from build123d import *

# Parameters (mm, degrees)
F0_R     = 43.75
F0_R_2   = 5
F1_DEPTH = 16
F2_R     = 7.5
F2_R_2   = 5
F3_DEPTH = 2.5
F4_R     = 39.3
F4_R_2   = 36.5
F4_R_3   = 32.8
F4_R_4   = 30
F5_DEPTH = 2.75
F6_SIZE  = 0.5


with BuildPart() as f1:
    # F0 (on Front) → F1 (new body)
    with BuildSketch(Plane.XZ):
        Circle(F0_R)
        Circle(F0_R_2, mode=Mode.SUBTRACT)
    extrude(amount=F1_DEPTH)

    # F2 (on face) → F3 (join)
    with BuildSketch(Plane.XZ.offset(16)):
        Circle(F2_R)
        Circle(F2_R_2, mode=Mode.SUBTRACT)
    extrude(amount=F3_DEPTH)

    # F4 (on face) → F5 (cut)
    with BuildSketch(Plane(origin=(0, 0, 0), x_dir=(-1, 0, 0), z_dir=(0, 1, 0))):
        Circle(F4_R)
        Circle(F4_R_2, mode=Mode.SUBTRACT)
        Circle(F4_R_3)
        Circle(F4_R_4, mode=Mode.SUBTRACT)
    extrude(amount=-F5_DEPTH, mode=Mode.SUBTRACT)

    # F6
    f6_edges = [f1.edges().sort_by_distance(p)[0] for p in [
        (-7.5, -18.5, 0),
        (-5, -18.5, 0),
        (-43.75, -16, 0),
        (-43.75, 0, 0),
        (-5, 0, 0),
    ]]
    chamfer(f6_edges, length=F6_SIZE)


solid = f1.part
The model under review builds one solid part; all positions refer to its coordinate system, in mm. A direction names the side the tool comes from. Give positions to 0.01 mm unless a question says otherwise; leave off trailing zeros. Write item = value, one per line. Start each with the question number.
(1) For L1, parallel to Z at x = 0, y = -1.8; L2, parallel to X at y = -2, z = 7.5; L3, parallel to Z at x = 0, y = -7.5, list the stretches that pass through material, from the lowest coordinate up. Write a range as from..to.
(2) For pin 1 Ø6 at (x, y) = (5, -13.5) entering from -Z; pin 2 Ø5 at (y, z) = (-8.5, 3) entering from -X; pin 3 Ø9 at (x, z) = (0, 0) entering from +Y; pin 4 Ø10 at (x, y) = (-16, -12) entering from -Z, all flat-tipped, find the tip position at first contact; note any pin that passes through.
(3) Tool access review of faces 4 (the cylindrical face through (4.27, -1.36, 32.52)), 5 (the cylindrical face through (-1.08, -9.13, -4.88)), 6 (the cylindrical face through (-7.493, -16.986, 0.33)): name each direction out of +Z, -Z, +X, -X, +Y, -Y from which nothing blocks a thin tool from reaching the whole face with its end or side.
(4) Draft analysis for pull direction X (two halves, no side actions). For faces 1 (the flat face through (-35, -2.75, -11)), 2 (the cylindrical face through (-32.246, -7.895, 29.568)), 3 (the flat face through (-30, 0, 14)), state which applies: +X half, -X half, draft (parallel to the pull), parting line (faces both ways), or undercut.
Returned:
q1.L1 = -43.75..-39.3, -36.5..-32.8, -30..-5, 5..30, 32.8..36.5, 39.3..43.75
q1.L2 = -43.1..-38.58, -35.72..-31.93, -29.05..29.05, 31.93..35.72, 38.58..43.1
q1.L3 = -43.75..-5, 5..43.75
q2.pin_1 = -43.7
q2.pin_2 = -43.75
q2.pin_3 = through
q2.pin_4 = -42.34
q3.face_4 = +Y
q3.face_5 = +Y, -Y
q3.face_6 = -Y
q4.face_1 = undercut
q4.face_2 = parting line
q4.face_3 = draft
